```python
from build123d import *

# Parameters (mm, degrees)
F0_W     = 50
F0_H     = 35
F1_DEPTH = 3
F2_D     = 6
F3_D     = 5
F4_D     = 5


with BuildPart() as f1:
    # F0 (on Top) → F1 (new body)
    with BuildSketch(Plane.XY):
        with Locations((-22.2067534924, 30.9401798017)):
            Rectangle(F0_W, F0_H)
    extrude(amount=F1_DEPTH)

    # F2 (through all)
    with Locations(Plane(origin=(0, 0, 0), x_dir=(1, 0, 0), z_dir=(0, 0, -1))):
        with Locations((-22.2067534924, -30.9401798017)):
            Hole(F2_D / 2)

    # F3 (through all)
    with Locations(Plane(origin=(0, 0, 0), x_dir=(1, 0, 0), z_dir=(0, 0, -1))):
        with Locations((-2.2067534924, -18.4401798017)):
            Hole(F3_D / 2)

    # F4 (through all)
    with Locations(Plane(origin=(0, 0, 0), x_dir=(1, 0, 0), z_dir=(0, 0, -1))):
        with Locations((-42.2067534924, -43.4401798017)):
            Hole(F4_D / 2)


solid = f1.part
```
Geometry: final body of the model. Coordinates: model frame, mm. Round coordinates to 2 decimals unless told otherwise and drop trailing zeros. Write each loop counter-clockwise with the first axis right and the second up, starting at its lowest first coordinate (ties: lowest second). Pieces come first, ordered by that corner, then holes. Notation, with made-up numbers: (83.5, -11) -> (93.5, -11) arc R36 ccw to (93.5, 24) -> close; hole circle Ø3 at (-9, 28). An arc over 180 degrees is marked (long way). Return JSON: item names as keys, results as strings.
Q1. Mould query, pull axis X, two halves, no side actions, for faces 1 (the flat face through (-47.207, 31, 1)), 2 (the cylindrical face through (-25.07, 30.04, 1.52)), 3 (the cylindrical face through (-1.88, 15.96, 1.52)), 4 (the flat face through (2.793, 31, 1)). Classes: +X half, -X half, draft (parallel to the pull), parting line (faces both ways), or undercut.
From the geometry:
{"face 1": "-X half", "face 2": "undercut", "face 3": "undercut", "face 4": "+X half"}
Q2. Section B-B on y = 45. Return the cut outline in (x, z), and give its area (3 significant figures).
From the geometry:
{"outline": "(-47.21, 0) -> (-44.16, 0) -> (-44.16, 3) -> (-47.21, 3) -> close; (-40.25, 0) -> (2.79, 0) -> (2.79, 3) -> (-40.25, 3) -> close", "area": "138 mm2"}
Q3. Ray query, line 1 (X direction, y = 42.5, z = 2.55); line 2 (X direction, y = 17.5, z = 0.75); line 3 (Y direction, x = -3, z = 0.45). Return the intervals inside material, ascending.
From the geometry:
{"line 1": "-47.21 to -44.52, -39.89 to 2.79", "line 2": "-47.21 to -4.52, 0.11 to 2.79", "line 3": "13.44 to 16.07, 20.81 to 48.44"}
Q4. Section A-A on z = 1.05. Return the cut outline in (x, y), and give its area (3 significant figures).
From the geometry:
{"outline": "(-47.21, 13.44) -> (2.79, 13.44) -> (2.79, 48.44) -> (-47.21, 48.44) -> close; hole circle Ø5 at (-42.21, 43.44); hole circle Ø6 at (-22.21, 30.94); hole circle Ø5 at (-2.21, 18.44)", "area": "1,680 mm2"}
Q5. Section C-C on y = 28.5. Return the cut outline in (x, z).
From the geometry:
{"outline": "(-47.21, 0) -> (-23.95, 0) -> (-23.95, 3) -> (-47.21, 3) -> close; (-20.46, 0) -> (2.79, 0) -> (2.79, 3) -> (-20.46, 3) -> close"}
